Input: part model. Units: mm. Frame: model coordinates. Face numbers are marked on the shaded views. A direction names the side the tool comes from. Coordinates: 2 decimals unless noted, no trailing zeros. Order: outer loops, then holes, each group sorted by start corner. A loop starts at its lowest first (then second) coordinate and runs counter-clockwise, first axis right, second up. Notation, with made-up numbers: (4, 66.25) - (10, 66.25) arc R21 cw to (10, 75.25) - close; hole circle Ø3 at (18, 41). An arc over 180 degrees is marked (long way). Use a Markdown table: item, result. Add a question column.
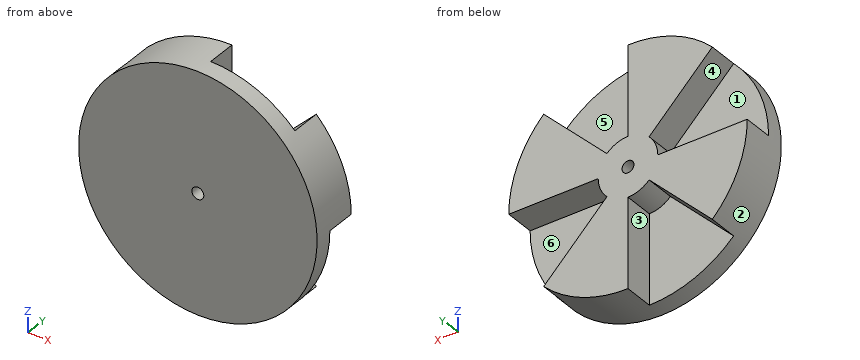
from build123d import *

# Parameters (mm, degrees)
SKETCH1_R                             = 20
EXTRUDE_MECHANISM_PART_2_DEPTH        = 8
CUT_START                             = -5
CUT_MECHANSIM_PART_2_DEPTH            = 5
SKETCH3_R                             = 1
HOLE_FOR_SCREW_MECHANSIM_PART_2_DEPTH = 10


with BuildPart() as part:
    # Sketch1 → Extrude (Mechanism Part 2) (new body)
    with BuildSketch(Plane(origin=(0, 0, 0), x_dir=(1, 0, 0), z_dir=(0, 1, 0))):
        with Locations(Location((0, 0, 0), (0, 0, 270))):
            Circle(SKETCH1_R)
    extrude(amount=EXTRUDE_MECHANISM_PART_2_DEPTH)

    # Sketch2 → Cut (Mechansim Part 2) (cut)
    with BuildSketch(Plane(origin=(0, 8, 0), x_dir=(1, 0, 0), z_dir=(0, 1, 0)).offset(CUT_START)):
        with BuildLine():
            ThreePointArc((-3.535533906, 3.535533906), (-1.913417162, 4.619397663), (0, 5))
            Line((0, 5), (0, 20))
            ThreePointArc((0, 20), (-7.653668647, 18.47759065), (-14.142135624, 14.142135624))
            Line((-14.142135624, 14.142135624), (-3.535533906, 3.535533906))
        make_face()
        with BuildLine():
            ThreePointArc((-3.535533906, -3.535533906), (-4.619397663, -1.913417162), (-5, 0))
            Line((-5, 0), (-20, 0))
            ThreePointArc((-20, 0), (-18.47759065, -7.653668647), (-14.142135624, -14.142135624))
            Line((-14.142135624, -14.142135624), (-3.535533906, -3.535533906))
        make_face()
        with BuildLine():
            ThreePointArc((3.535533906, -3.535533906), (1.913417162, -4.619397663), (0, -5))
            Line((0, -5), (0, -20))
            ThreePointArc((0, -20), (7.653668647, -18.47759065), (14.142135624, -14.142135624))
            Line((14.142135624, -14.142135624), (3.535533906, -3.535533906))
        make_face()
        with BuildLine():
            ThreePointArc((3.535533906, 3.535533906), (4.619397663, 1.913417162), (5, 0))
            Line((5, 0), (20, 0))
            ThreePointArc((20, 0), (18.47759065, 7.653668647), (14.142135624, 14.142135624))
            Line((14.142135624, 14.142135624), (3.535533906, 3.535533906))
        make_face()
    extrude(amount=CUT_MECHANSIM_PART_2_DEPTH, mode=Mode.SUBTRACT)

    # Sketch3 → Hole for Screw (Mechansim Part 2) (cut)
    with BuildSketch(Plane(origin=(0, 8, 0), x_dir=(1, 0, 0), z_dir=(0, 1, 0))):
        with Locations(Location((0, 0, 0), (0, 0, 270))):
            Circle(SKETCH3_R)
    extrude(amount=-HOLE_FOR_SCREW_MECHANSIM_PART_2_DEPTH, mode=Mode.SUBTRACT)


solid = part.part
1) Reachability of the marked faces 4, 5 and 6 from +Z, -Z, +X, -X, +Y, -Y: full face, straight path, thin tool, end or side. Return the list, or none.
2) Pull-direction query (X, two-part tool) for the marked faces 1, 2 and 3; classes: pulls with the +X half, pulls with the -X half, needs draft (parallel to the pull), parting line crosses it, or undercut.
3) Cut plane C-C (x = -11). Return the cut outline in (y, z), and give its area (3 significant figures).
4) Cut plane B-B (z = -11). Return the cut outline in (x, y).
5) Material intervals for L1, parallel to X at y = 3.5, z = -8; L2, parallel to Z at x = -14, y = 7.75; L3, parallel to Y at x = 2.5, z = 9, sorted ascending.
6) Cut plane A-A (y = 5.25). Return the cut outline in (x, z).
7) Contact query for flat-ended pins moving along their axis: P1, Ø2.5, axis at x = 13.5, y = 6.5, coming from the -Z side; P2, Ø1.5, axis at x = -11, y = 4.5, coming from the +Z side; P3, Ø3, axis at y = 5, z = -5.5, coming from the +X side. Output: stop coordinate, or through.
8) Cut plane D-D (z = 16). Return the cut outline in (x, y).
Computed:
| question | item | result |
|---|---|---|
| 1 | face 4 | -X, +Y |
| 1 | face 5 | +Z, +Y |
| 1 | face 6 | +X, +Y |
| 2 | face 1 | needs draft |
| 2 | face 2 | parting line crosses it |
| 2 | face 3 | undercut |
| 3 | outline | (0, -16.7) - (3, -16.7) - (3, -11) - (8, -11) - (8, 0) - (3, 0) - (3, 11) - (8, 11) - (8, 16.7) - (0, 16.7) - close |
| 3 | area | 184 mm2 |
| 4 | outline | (-16.7, 0) - (16.7, 0) - (16.7, 3) - (11, 3) - (11, 8) - (0, 8) - (0, 3) - (-11, 3) - (-11, 8) - (-16.7, 8) - close |
| 5 | L1 | x = -18.33 to -8, 0 to 8 |
| 5 | L2 | z = -14 to 0, 14 to 14.28 |
| 5 | L3 | y = 0 to 3 |
| 6 | outline | (-20, 0) arc R20 ccw to (-14.14, -14.14) - (-3.54, -3.54) arc R5 ccw to (0, -5) - (0, -20) arc R20 ccw to (14.14, -14.14) - (3.54, -3.54) arc R5 ccw to (5, 0) - (20, 0) arc R20 ccw to (14.14, 14.14) - (3.54, 3.54) arc R5 ccw to (0, 5) - (0, 20) arc R20 ccw to (-14.14, 14.14) - (-3.54, 3.54) arc R5 ccw to (-5, 0) - close; hole circle Ø2 at (0, 0) |
| 7 | P1 | stops at z = -15.81 |
| 7 | P2 | stops at z = 17.17 |
| 7 | P3 | stops at x = 7 |
| 8 | outline | (-12, 0) - (12, 0) - (12, 3) - (0, 3) - (0, 8) - (-12, 8) - close |
